Drawing for the job (mm, zero at the part's lowest x, y, z). Round coordinates to 2 decimals unless told otherwise and drop trailing zeros. Order: outer loops, then holes, each group sorted by start corner. A loop starts at its lowest first (then second) coordinate and runs counter-clockwise, first axis right, second up. Notation, with made-up numbers: M 25,74 L 65,74 A7 ccw 65,83 Z; hole C 45.25,59.5 d6. An arc over 180 degrees is marked long. One line per item, written item: value. Start each with the question number.
Item 1: Band-saw the part on A-A, the plane y = 21. Write the cut outline in (x, z) (1 decimal).
Item 2: Pin check, flat tips, straight feed: pin 1 (8 mm diameter, centred on x = 43.5, y = 6.5, fed in from -Z) (1 decimal); pin 2 (6 mm diameter, centred on y = 4, z = 56.5, fed in from +X) (1 decimal); pin 3 (4 mm diameter, centred on y = 3, z = 30, fed in from -X). Stop position of each tip, or through.
Item 3: Band-saw the part on C-C, the plane z = 15.5. Write the cut outline in (x, y), then the cut area to 3 significant figures.
Item 4: Band-saw the part on B-B, the plane x = 30.5. Write the cut outline in (y, z), then the cut area to 3 significant figures.
Item 5: Probe L1, parallel to Z at x = 47.5, y = 17.25 (1 decimal); L2, parallel to X at y = 8.75, z = 61 (1 decimal); L3, parallel to X at y = 7.5, z = 60.5 (1 decimal). List the from-to ranges inside material, lowest first.
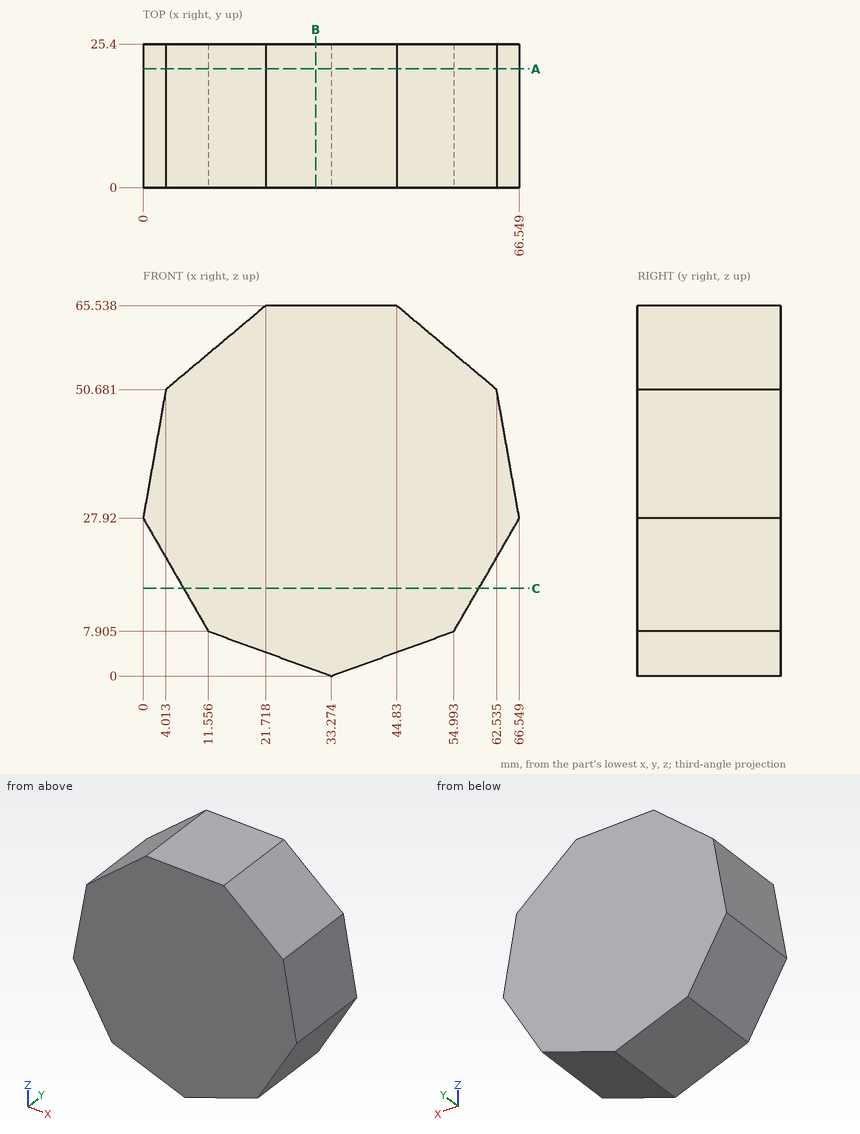
Output:
1. outline: M 0,27.9 L 11.6,7.9 L 33.3,0 L 55,7.9 L 66.5,27.9 L 62.5,50.7 L 44.8,65.5 L 21.7,65.5 L 4,50.7 Z
2. pin 1: stops at z = 2.3
2. pin 2: stops at x = 59.2
2. pin 3: stops at x = 0.01
3. outline: M 7.17,0 L 59.38,0 L 59.38,25.4 L 7.17,25.4 Z
3. area: 1,330 mm²
4. outline: M 0,1.01 L 25.4,1.01 L 25.4,65.54 L 0,65.54 Z
4. area: 1,640 mm²
5. L1: z = 5.2 to 63.3
5. L2: x = 16.3 to 50.2
5. L3: x = 15.7 to 50.8
